Geometry check sheet. Reference: the model listing, model coordinates, mm. A direction names the side the tool comes from. Round coordinates to 2 decimals unless told otherwise and drop trailing zeros. Order: outer loops, then holes, each group sorted by start corner. A loop starts at its lowest first (then second) coordinate and runs counter-clockwise, first axis right, second up. Notation, with made-up numbers: (22.25, 23) -> (48.25, 23) arc R23 ccw to (48.25, 38) -> close; hole circle Ø10 at (-8, 6.5). An arc over 180 degrees is marked (long way). Answer as a JSON object with one key per item and string values. Group by question number.
from build123d import *

# Parameters (mm, degrees)
SKETCH1_W           = 8.3
SKETCH1_H           = 9.8906033
BOSS_EXTRUDE1_DEPTH = 9
SKETCH2_W           = 10
SKETCH2_H           = 3.6906033
BOSS_EXTRUDE2_DEPTH = 9


with BuildPart() as part:
    # Sketch1 → Boss-Extrude1 (new body)
    with BuildSketch(Plane.XY):
        with Locations((4.15, 4.94530165)):
            Rectangle(SKETCH1_W, SKETCH1_H)
    extrude(amount=BOSS_EXTRUDE1_DEPTH)

    # Sketch2 → Boss-Extrude2 (add, through all)
    with BuildSketch(Plane.XY.offset(9)):
        with Locations((13.3, 8.04530165)):
            Rectangle(SKETCH2_W, SKETCH2_H)
        with Locations((13.3, 3.15469835)):
            Rectangle(SKETCH2_W, SKETCH2_H)
    extrude(amount=-BOSS_EXTRUDE2_DEPTH)


solid = part.part
Item 1: Set-up check for faces 1 (the flat face through (13, 5, 5)), 2 (the flat face through (4, 0, 4)), 3 (the flat face through (13, 1.309, 5)): record each of +Z, -Z, +X, -X, +Y, -Y from which the full face is reachable in a straight line by a thin tool's end or side.
Item 2: Thickness scan on L1, parallel to Y at x = 9, z = 6; L2, parallel to X at y = 0.5, z = 7.25. Record the ranges inside material, lowest first.
Item 3: Mould release check, pull along Y, two halves, no side actions. Record for faces 4 (the flat face through (9, 9.891, 5)), 5 (the flat face through (8.3, 6, 4)), 6 (the flat face through (13, 6.2, 5)), 7 (the flat face through (7, 5, 0)): pulls with the +Y half, pulls with the -Y half, needs draft (parallel to the pull), parting line crosses it, or undercut.
Item 4: Sectioned sample at B-B, the plane z = 3. Enter the section's corners in (x, y).
Item 5: Sectioned sample at A-A, the plane x = 14.75. Enter the section's corners in (y, z).
Item 6: Depth check by flat-ended pin: pin 1 Ø0.7 at (y, z) = (0.5, 5.5) entering from +X; pin 2 Ø4.5 at (x, z) = (11, 4) entering from -Y. Enter the tip coordinate at first touch or a pass-through.
Result:
{
 "1": {"face 1": "+Z, -Z, +X", "face 2": "+Z, -Z, +X, -X, -Y", "face 3": "+Z, -Z, +X, -Y"},
 "2": {"L1": "y = 1.31 to 5, 6.2 to 9.89", "L2": "x = 0 to 8.3"},
 "3": {"face 4": "pulls with the +Y half", "face 5": "undercut", "face 6": "undercut", "face 7": "needs draft"},
 "4": {"outline": "(0, 0) -> (8.3, 0) -> (8.3, 1.31) -> (18.3, 1.31) -> (18.3, 5) -> (8.3, 5) -> (8.3, 6.2) -> (18.3, 6.2) -> (18.3, 9.89) -> (0, 9.89) -> close"},
 "5": {"outline": "(1.31, 0) -> (5, 0) -> (5, 9) -> (1.31, 9) -> close; (6.2, 0) -> (9.89, 0) -> (9.89, 9) -> (6.2, 9) -> close"},
 "6": {"pin 1": "stops at x = 8.3", "pin 2": "stops at y = 1.31"}
}
